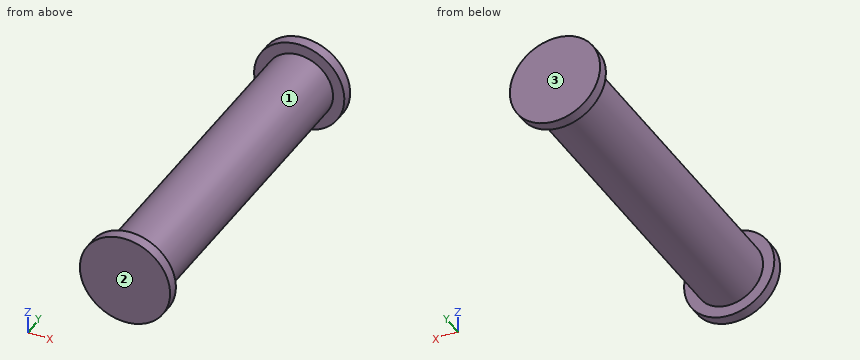
from build123d import *

# Parameters (mm, degrees)
SKETCH1_R           = 3
BOSS_EXTRUDE1_DEPTH = 30
SKETCH2_R           = 4
BOSS_EXTRUDE2_DEPTH = 1
SKETCH3_R           = 4
BOSS_EXTRUDE3_DEPTH = 1


with BuildPart() as part:
    # Sketch1 → Boss-Extrude1 (new body)
    with BuildSketch(Plane(origin=(0, 0, 0), x_dir=(1, 0, 0), z_dir=(0, 1, 0))):
        with Locations(Location((0, 0, 0), (0, 0, 270))):
            Circle(SKETCH1_R)
    extrude(amount=-BOSS_EXTRUDE1_DEPTH)

    # Sketch2 → Boss-Extrude2 (add)
    with BuildSketch(Plane(origin=(0, 0, 0), x_dir=(1, 0, 0), z_dir=(0, 1, 0))):
        with Locations(Location((0, 0, 0), (0, 0, 270))):
            Circle(SKETCH2_R)
    extrude(amount=-BOSS_EXTRUDE2_DEPTH)

    # Sketch3 → Boss-Extrude3 (add)
    with BuildSketch(Plane.XZ.offset(30)):
        with Locations(Location((0, 0, 0), (0, 0, 90))):
            Circle(SKETCH3_R)
    extrude(amount=BOSS_EXTRUDE3_DEPTH)


solid = part.part
Verification items for the finished model (mm, model axes). Face numbers are marked on the shaded views. Give positions to 0.01 mm unless a question says otherwise; leave off trailing zeros. Write each loop counter-clockwise with the first axis right and the second up, starting at its lowest first coordinate (ties: lowest second). Pieces come first, ordered by that corner, then holes. Notation, with made-up numbers: (69.25, -23.5) - (95.25, -23.5) arc R21 cw to (95.25, 13.5) - close; hole circle Ø3 at (23, 82). An arc over 180 degrees is marked (long way). Answer as CSV lines item,"result". Start each with the question number.
1. Sectioned sample at B-B (x = 0). Record the boundary of the cut face in (y, z), then the cut area to 3 significant figures.
2. Thickness scan on line 1 (Y direction, x = -2, z = -2.5); line 2 (X direction, y = -17, z = 0); line 3 (Z direction, x = -0.5, y = -22). Record the ranges inside material, lowest first.
3. Draft check along Y on the marked faces 1, 2 and 3. Enter one of: pulls with the +Y half, pulls with the -Y half, needs draft (parallel to the pull), parting line crosses it, or undercut.
4. Depth check by flat-ended pin: pin 1 (1.5 mm diameter, centred on x = -1.5, y = -5.5, fed in from -Z); pin 2 (3 mm diameter, centred on x = -0.5, y = -24.5, fed in from -Z); pin 3 (4 mm diameter, centred on y = -24, z = -2.5, fed in from -X). Enter the tip coordinate at first touch or a pass-through.
5. Sectioned sample at C-C (y = -10.5). Record the boundary of the cut face in (x, z), then the cut area to 3 significant figures.
6. Sectioned sample at A-A (z = 0). Record the boundary of the cut face in (x, y).
Derived:
1,outline,"(-31, -4) - (-30, -4) - (-30, -3) - (-1, -3) - (-1, -4) - (0, -4) - (0, 4) - (-1, 4) - (-1, 3) - (-30, 3) - (-30, 4) - (-31, 4) - close"
1,area,"190 mm²"
2,line 1,"-31 to -30, -1 to 0"
2,line 2,"-3 to 3"
2,line 3,"-2.96 to 2.96"
3,face 1,"undercut"
3,face 2,"pulls with the -Y half"
3,face 3,"pulls with the +Y half"
4,pin 1,"z = -2.9"
4,pin 2,"z = -3"
4,pin 3,"x = -2.96"
5,outline,"circle Ø6 at (0, 0)"
5,area,"28.3 mm²"
6,outline,"(-4, -31) - (4, -31) - (4, -30) - (3, -30) - (3, -1) - (4, -1) - (4, 0) - (-4, 0) - (-4, -1) - (-3, -1) - (-3, -30) - (-4, -30) - close"
